from build123d import *

# Parameters (mm, degrees)
ESQUISSE1_R             = 20
BOSS_EXTRU_1_DEPTH      = 20
ESQUISSE1_R_2           = 60
ESQUISSE1_R_3           = 50
BOSS_EXTRU_1_2_DEPTH    = 20
ESQUISSE2_R             = 50
ESQUISSE2_R_2           = 20
BOSS_EXTRU_2_DEPTH      = 10
CHANFREIN1_SIZE         = 5
CONG_1_R                = 5
ESQUISSE3_R             = 10
ENL_V_MAT_EXTRU_1_DEPTH = 82


with BuildPart() as part:
    # Esquisse1 → Boss.-Extru.1 (new body)
    with BuildSketch(Plane(origin=(0, 0, 0), x_dir=(1, 0, 0), z_dir=(0, 1, 0))):
        with Locations((24.301532902, 9.851972798)):
            Circle(ESQUISSE1_R)
    extrude(amount=BOSS_EXTRU_1_DEPTH)



with BuildPart() as body_2:
    # Esquisse1 → Boss.-Extru.1 2 (new body)
    with BuildSketch(Plane(origin=(0, 0, 0), x_dir=(1, 0, 0), z_dir=(0, 1, 0))):
        with Locations((24.301532902, 9.851972798)):
            Circle(ESQUISSE1_R_2)
        with Locations((24.301532902, 9.851972798)):
            Circle(ESQUISSE1_R_3, mode=Mode.SUBTRACT)
    extrude(amount=BOSS_EXTRU_1_2_DEPTH)


with BuildPart() as part_1:
    add(part.part)

    add(body_2.part)  # Boss.-Extru.2 merges body 2
    # Esquisse2 → Boss.-Extru.2 (add)
    with BuildSketch(Plane.XZ):
        with Locations((24.301532902, -9.851972798)):
            Circle(ESQUISSE2_R)
        with Locations((24.301532902, -9.851972798)):
            Circle(ESQUISSE2_R_2, mode=Mode.SUBTRACT)
    extrude(amount=-BOSS_EXTRU_2_DEPTH)

    # Chanfrein1
    chanfrein1_edges = [part_1.edges().sort_by_distance(p)[0] for p in [
        (-25.698467098, 20, -9.851972798),
    ]]
    chamfer(chanfrein1_edges, length=CHANFREIN1_SIZE)

    # Congé1
    cong_1_edges = [part_1.edges().sort_by_distance(p)[0] for p in [
        (4.301532902, 20, -9.851972798),
    ]]
    fillet(cong_1_edges, radius=CONG_1_R)

    # Esquisse3 → Enlèv. mat.-Extru.1 (cut)
    with BuildSketch(Plane(origin=(0, 20, 0), x_dir=(1, 0, 0), z_dir=(0, 1, 0))):
        with Locations((24.301532902, 9.851972798)):
            Circle(ESQUISSE3_R)
    extrude(amount=-ENL_V_MAT_EXTRU_1_DEPTH, mode=Mode.SUBTRACT)


solid = part_1.part
Here's how the part is built. I have some questions about the finished solid (model axes, mm). A direction names the side the tool comes from. Coordinates: 2 decimals unless noted, no trailing zeros. Write each loop counter-clockwise with the first axis right and the second up, starting at its lowest first coordinate (ties: lowest second). Pieces come first, ordered by that corner, then holes.
Item 1: Will these pins go through, and if not, where does the flat tip stop? pin 1 (2 mm diameter, centred on y = 17, z = -30, fed in from -X); pin 2 (3 mm diameter, centred on x = -10, z = -2.5, fed in from +Y); pin 3 (10 mm diameter, centred on y = 11.5, z = -23, fed in from -X).
Item 2: I want a section at A-A on y = 13. Write out the boundary of the cut face in (x, z), and give its area (3 significant figures).
Item 3: I want a section at B-B on y = 7. Write out the boundary of the cut face in (x, z), and give its area (3 significant figures).
Item 4: If we mould it in two halves opening along Z, with no side actions, what happens to faces 1 (the flat face through (51, 20, 39)), 2 (the conical face through (47.486, 15.243, 34.722)), 3 (the flat face through (46, 10, -9)), 4 (the cylindrical face through (79.726, 9.86, 13.128))? For each: +Z half, -Z half, draft (parallel to the pull), parting line (faces both ways), or undercut.
Item 5: If I drill on line 1 (X direction, y = 15, z = -20.5); line 2 (X direction, y = 16.75, z = 31); line 3 (Y direction, x = 11.5, z = 6.5), over which ranges is the centre line in solid material (lowest first)?
Item 6: On a 3-axis mill with a long thin cutter (end or side, diameter ignored), from which of +Z, -Z, +X, -X, +Y, -Y can I reach the whole of each face in a straight line? I mean faces 5 (the cylindrical face through (-15.38, 12.46, 20.57)), 6 (the flat face through (37, 0, -9)). Say none if no direction works.
Findings below:
1. pin 1: stops at x = -32.56
1. pin 2: stops at y = 10
1. pin 3: stops at x = -35.14
2. outline: circle Ø120 at (24.3, -9.85); circle Ø40 at (24.3, -9.85); hole circle Ø100 at (24.3, -9.85); hole circle Ø20 at (24.3, -9.85)
2. area: 4,400 mm2
3. outline: circle Ø120 at (24.3, -9.85); hole circle Ø20 at (24.3, -9.85)
3. area: 11,000 mm2
4. face 1: draft
4. face 2: undercut
4. face 3: undercut
4. face 4: parting line
5. line 1: x = -34.75 to -24.55, 7.37 to 41.23, 73.15 to 83.35
5. line 2: x = -19.64 to -7.47, 56.07 to 68.25
5. line 3: y = 0 to 10
6. face 5: +Y
6. face 6: +Z, -Z, +X, -X, -Y
